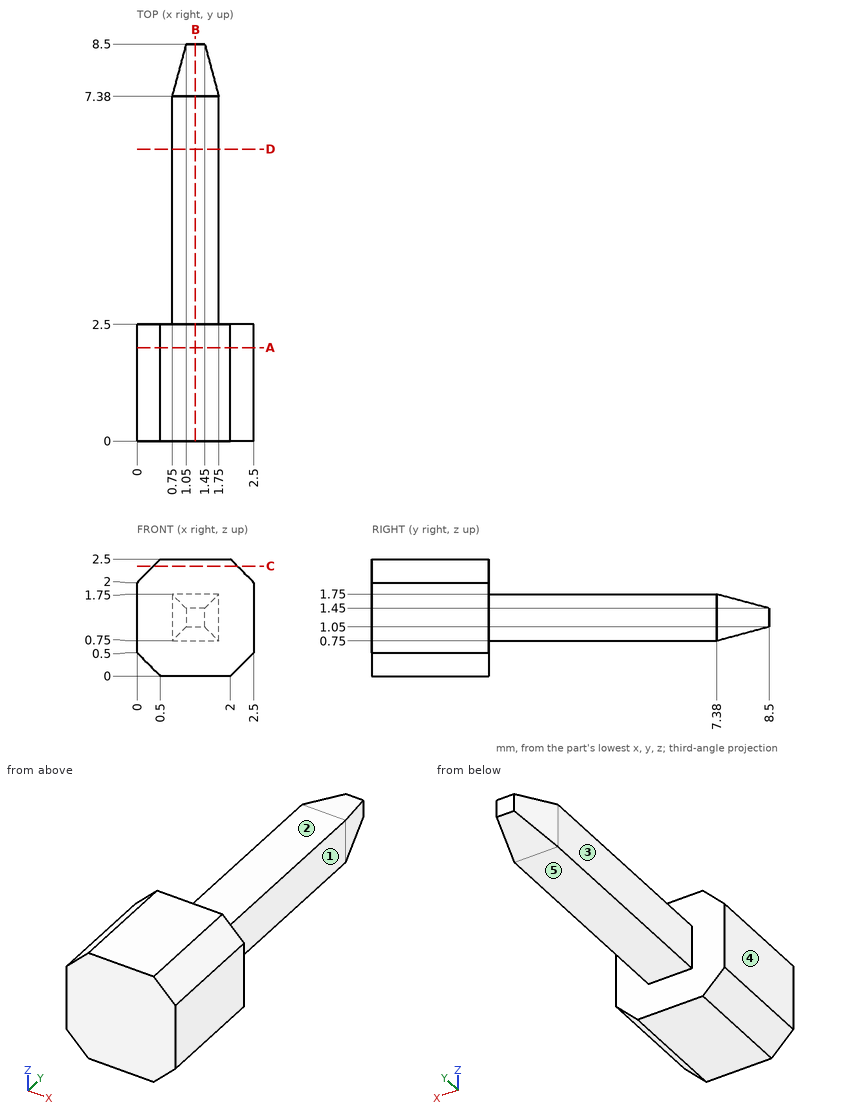
Geometry: see drawing. Coordinates: mm, zero at the bounding-box minimum. A direction names the side the tool comes from. Coordinates: 2 decimals unless noted, no trailing zeros. Order: outer loops, then holes, each group sorted by start corner. A loop starts at its lowest first (then second) coordinate and runs counter-clockwise, first axis right, second up. Notation, with made-up numbers: M 75,85 L 87,85 A12 cw 87,98 Z; hole C 77.5,64 d8. An arc over 180 degrees is marked long. Answer in a Markdown table with one row per item. Add a question column.
Q1. Section query A-A on y = 2. Return the cut outline in (x, z).
Q2. Section query D-D on y = 6.25. Return the cut outline in (x, z).
Q3. Contact query for flat-ended pins moving along their axis: P1, Ø0.5, axis at y = 5.5, z = 1, coming from the -X side; P2, Ø0.5, axis at y = 5.5, z = 1, coming from the +X side; P3, Ø1.1, axis at x = 1.5, y = 5, coming from the +Z side. Output: stop coordinate, or through.
Q4. Line query: L1, parallel to Y at x = 1.75, z = 2.2; L2, parallel to X at y = 3.25, z = 1.2; L3, parallel to X at y = 7.5, z = 0.85. Output: solid intervals per line, ascending.
Q5. Section query B-B on x = 1.25. Return the cut outline in (y, z), and give its area (3 significant figures).
Q6. Reachability of the marked faces 1, 2, 3, 4 and 5 from +Z, -Z, +X, -X, +Y, -Y: full face, straight path, thin tool, end or side. Return the list, or none.
Q7. Section query C-C on z = 2.35. Return the cut outline in (x, y).
Completed:
| question | item | result |
|---|---|---|
| 1 | outline | M 0,0.5 L 0.5,0 L 2,0 L 2.5,0.5 L 2.5,2 L 2,2.5 L 0.5,2.5 L 0,2 Z |
| 2 | outline | M 0.75,0.75 L 1.75,0.75 L 1.75,1.75 L 0.75,1.75 Z |
| 3 | P1 | stops at x = 0.75 |
| 3 | P2 | stops at x = 1.75 |
| 3 | P3 | stops at z = 1.75 |
| 4 | L1 | y = 0 to 2.5 |
| 4 | L2 | x = 0.75 to 1.75 |
| 4 | L3 | x = 0.78 to 1.72 |
| 5 | outline | M 0,0 L 2.5,0 L 2.5,0.75 L 7.38,0.75 L 8.5,1.05 L 8.5,1.45 L 7.38,1.75 L 2.5,1.75 L 2.5,2.5 L 0,2.5 Z |
| 5 | area | 11.9 mm2 |
| 6 | face 1 | +Z, -Z, +X, +Y |
| 6 | face 2 | +Z, +X, -X, +Y |
| 6 | face 3 | +Z, -Z, -X, +Y |
| 6 | face 4 | +Z, -Z, -X, +Y, -Y |
| 6 | face 5 | -Z, +X, -X, +Y |
| 7 | outline | M 0.35,0 L 2.15,0 L 2.15,2.5 L 0.35,2.5 Z |
